```python
from build123d import *

# Parameters (mm, degrees)
SKETCH1_W           = 109.5
SKETCH1_H           = 14.5
BOSS_EXTRUDE5_DEPTH = 15
BOSS_EXTRUDE6_DEPTH = 9.5
BOSS_EXTRUDE8_DEPTH = 13
SKETCH4_W           = 6.5
SKETCH4_H           = 11.5
CUT_EXTRUDE3_DEPTH  = 65.5
FILLET2_R           = 2.5


with BuildPart() as part:
    # Sketch1 → Boss-Extrude5 (new, symmetric)
    with BuildSketch(Plane(origin=(0, 0, 0), x_dir=(1, 0, 0), z_dir=(0, 1, 0))):
        with Locations((54.75, -40.75)):
            Rectangle(SKETCH1_W, SKETCH1_H)
    extrude(amount=BOSS_EXTRUDE5_DEPTH, both=True)

    # Sketch1<3> → Boss-Extrude6 (add, symmetric)
    with BuildSketch(Plane(origin=(0, 0, 0), x_dir=(1, 0, 0), z_dir=(0, 1, 0))):
        Polygon((105, 0), (0, 0), (0, -33.5), (109.5, -33.5), (116.5, -33.5), (133, -17), (105, -17), align=None)
        with BuildLine():
            ThreePointArc((30.5, -23), (25, -17.5), (30.5, -12))
            Line((30.5, -12), (81.5, -12))
            ThreePointArc((81.5, -12), (87, -17.5), (81.5, -23))
            Line((81.5, -23), (30.5, -23))
        make_face(mode=Mode.SUBTRACT)
    extrude(amount=BOSS_EXTRUDE6_DEPTH, both=True)

    # Sketch1<5> → Boss-Extrude8 (add, symmetric)
    with BuildSketch(Plane(origin=(0, 0, 0), x_dir=(1, 0, 0), z_dir=(0, 1, 0))):
        Polygon((140, 0), (105, 0), (105, -17), (133, -17), (140, -10), align=None)
    extrude(amount=BOSS_EXTRUDE8_DEPTH, both=True)

    # Sketch4 → Cut-Extrude3 (cut, symmetric)
    with BuildSketch(Plane(origin=(0, 0, 0), x_dir=(-1, 0, 0), z_dir=(0, 0, -1))):
        with Locations((-3.25, 9.25)):
            Rectangle(SKETCH4_W, SKETCH4_H)
    extrude(amount=CUT_EXTRUDE3_DEPTH, both=True, mode=Mode.SUBTRACT)

    # Fillet2
    fillet2_edges = [part.edges().sort_by_distance(p)[0] for p in [
        (87, 9.5, 17.5),
        (56, 9.5, 23),
        (25, 9.5, 17.5),
        (56, -9.5, 12),
        (56, 9.5, 12),
        (87, -9.5, 17.5),
        (25, -9.5, 17.5),
        (56, -9.5, 23),
    ]]
    fillet(fillet2_edges, radius=FILLET2_R)

    # Mirror2: part across plane


with BuildPart() as part_1:
    add(part.part)
    add(part.part.mirror(Plane(origin=(0, 15, 48), x_dir=(1, 0, 0), z_dir=(0, 0, -1))))


solid = part_1.part
```
Input: part model. Units: mm. Frame: model coordinates. A direction names the side the tool comes from. Round coordinates to 2 decimals unless told otherwise and drop trailing zeros. Order: outer loops, then holes, each group sorted by start corner. A loop starts at its lowest first (then second) coordinate and runs counter-clockwise, first axis right, second up. Notation, with made-up numbers: (-24.5, 21.25) - (6.5, 21.25) arc R13 ccw to (6.5, 28.25) - close; hole circle Ø11 at (41.25, 25.5). An arc over 180 degrees is marked (long way). One line per question, with ' | ' between items. Start each with the question number.
1) Pull-direction query (X, two-part tool) for faces 5 (the flat face through (119, -11, 79)), 6 (the flat face through (56, 0, 84)), 7 (the flat face through (105, 11, 88)); classes: +X half, -X half, draft (parallel to the pull), parting line (faces both ways), or undercut.
2) Cut plane C-C, the plane y = 0.25. Return the cut outline in (x, z).
3) Ray query, probe 1 along Z at (x, y) = (107, 12.75); probe 2 along Z at (x, y) = (33, -0.25); probe 3 along Z at (x, y) = (100, 13.5). Return the intervals inside material, ascending.
4) Contact query for flat-ended pins moving along their axis: P1, Ø3, axis at x = 112.5, y = -10.5, coming from the -Z side; P2, Ø6, axis at y = 9, z = 31.5, coming from the -X side; P3, Ø5, axis at y = -10.5, z = 57, coming from the +X side; P4, Ø8.5, axis at x = 116.5, z = 90, coming from the +Y side. Output: stop coordinate, or through.
5) Cut plane A-A, the plane x = 40.5. Return the cut outline in (y, z), then the cut area to 3 significant figures.
6) Cut plane B-B, the plane z = 61. Return the cut outline in (x, y), then the cut area to 3 significant figures.
7) Cut plane D-D, the plane x = 113. Return the cut outline in (y, z), then the cut area to 3 significant figures.
8) Set-up query: faces 1 (the flat face through (128, 0, 74)), 2 (the flat face through (54, -15, 48)), 3 (the cylindrical face through (87, 0.1, 17.4)), 4 (the flat face through (119, 11, 79)). Return all of +Z, -Z, +X, -X, +Y, -Y with unobstructed straight access to the full face (end or side cutting, diameter ignored); none if empty.
Worked out:
1) face 5: draft | face 6: undercut | face 7: -X half
2) outline: (0, 0) - (140, 0) - (140, 10) - (116.5, 33.5) - (109.5, 33.5) - (109.5, 62.5) - (116.5, 62.5) - (140, 86) - (140, 96) - (0, 96) - close; hole (30.5, 12) - (81.5, 12) arc R5.5 ccw to (81.5, 23) - (30.5, 23) arc R5.5 ccw to start; hole (30.5, 73) - (81.5, 73) arc R5.5 ccw to (81.5, 84) - (30.5, 84) arc R5.5 ccw to start
3) probe 1: z = 0 to 17, 33.5 to 62.5, 79 to 96 | probe 2: z = 0 to 12, 23 to 73, 84 to 96 | probe 3: z = 33.5 to 62.5
4) P1: stops at z = 0 | P2: stops at x = 6.5 | P3: stops at x = 109.5 | P4: stops at y = 13
5) outline: (-15, 33.5) - (-9.5, 33.5) - (-9.5, 25.5) arc R2.5 ccw to (-7, 23) - (7, 23) arc R2.5 ccw to (9.5, 25.5) - (9.5, 33.5) - (15, 33.5) - (15, 62.5) - (9.5, 62.5) - (9.5, 70.5) arc R2.5 ccw to (7, 73) - (-7, 73) arc R2.5 ccw to (-9.5, 70.5) - (-9.5, 62.5) - (-15, 62.5) - close; (-9.5, 0) - (9.5, 0) - (9.5, 9.5) arc R2.5 ccw to (7, 12) - (-7, 12) arc R2.5 ccw to (-9.5, 9.5) - close; (-9.5, 86.5) arc R2.5 ccw to (-7, 84) - (7, 84) arc R2.5 ccw to (9.5, 86.5) - (9.5, 96) - (-9.5, 96) - close | area: 1,710 mm^2
6) outline: (0, -15) - (109.5, -15) - (109.5, 15) - (6.5, 15) - (6.5, 3.5) - (0, 3.5) - close | area: 3,210 mm^2
7) outline: (-13, 0) - (13, 0) - (13, 17) - (9.5, 17) - (9.5, 33.5) - (-9.5, 33.5) - (-9.5, 17) - (-13, 17) - close; (-13, 79) - (-9.5, 79) - (-9.5, 62.5) - (9.5, 62.5) - (9.5, 79) - (13, 79) - (13, 96) - (-13, 96) - close | area: 1,510 mm^2
8) face 1: +X, +Y, -Y | face 2: +Z, -Z, +X, -X, -Y | face 3: +Y, -Y | face 4: +X, -X, +Y
